The listing builds one solid part. Answer for the finished solid, in the listing's coordinates (mm). Face numbers are marked on the shaded views. A direction names the side the tool comes from. Coordinates: 2 decimals unless noted, no trailing zeros. Write each loop counter-clockwise with the first axis right and the second up, starting at its lowest first coordinate (ties: lowest second). Pieces come first, ordered by that corner, then holes. Notation, with made-up numbers: M 80.25,60 L 124.25,60 A21 ccw 124.25,93 Z; hole C 68,61 d4. An arc over 180 degrees is marked long. Answer as a JSON object with one key per item and string values. Group by question number.
from build123d import *

# Parameters (mm, degrees)
SKETCH_1_W                    = 120
SKETCH_1_H                    = 40
EXTRUDE_1_DEPTH               = 14
SKETCH_2_W                    = 120
SKETCH_2_H                    = 20
CUT_EXTRUDE_1_DEPTH           = 2
HOLE_WIZARD_M12_1_D           = 13.5
HOLE_WIZARD_M12_1_CBORE_D     = 20
HOLE_WIZARD_M12_1_CBORE_DEPTH = 10
FILLET_1_R                    = 20
HOLE_WIZARD_M6_1_D            = 5


with BuildPart() as part:
    # 草图1 → 凸台-拉伸1 (new body)
    with BuildSketch(Plane.XY):
        Rectangle(SKETCH_1_W, SKETCH_1_H)
    extrude(amount=EXTRUDE_1_DEPTH)

    # 草图2 → 切除-拉伸1 (cut)
    with BuildSketch(Plane.XY.offset(14)):
        Rectangle(SKETCH_2_W, SKETCH_2_H)
    extrude(amount=-CUT_EXTRUDE_1_DEPTH, mode=Mode.SUBTRACT)

    # M12 六角头螺栓的柱形沉头孔1 (through all)
    with Locations(Plane.XY.offset(12)):
        with Locations((-35, 0), (35, 0)):
            CounterBoreHole(HOLE_WIZARD_M12_1_D / 2, HOLE_WIZARD_M12_1_CBORE_D / 2, HOLE_WIZARD_M12_1_CBORE_DEPTH)

    # 圆角1
    fillet_1_edges = [part.edges().sort_by_distance(p)[0] for p in [
        (60, 20, 7),
        (60, -20, 7),
        (-60, -20, 7),
        (-60, 20, 7),
    ]]
    fillet(fillet_1_edges, radius=FILLET_1_R - 0.0001)  # a hair under: the kernel refuses the full size

    # M6 螺纹孔1 (through all)
    with Locations(Plane.XY.offset(12)):
        with Locations((0, 0)):
            Hole(HOLE_WIZARD_M6_1_D / 2)


solid = part.part
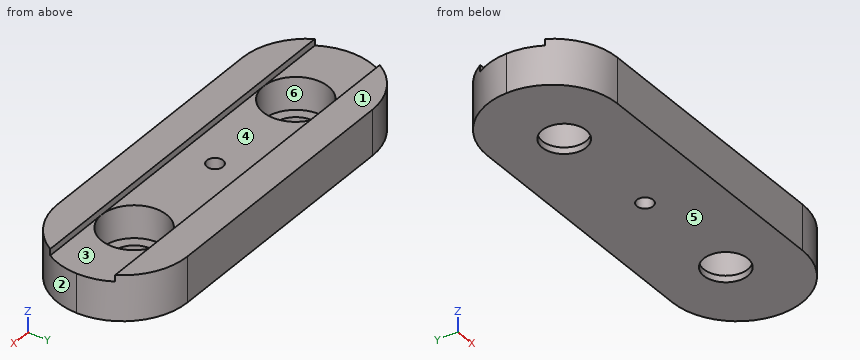
Item 1: Consider L1, parallel to Y at x = 35, z = 1; L2, parallel to X at y = -1, z = 11.25; L3, parallel to Y at x = -35, z = 8.75. Determine where each line is inside the solid, lowest interval first. Write a range as from..to.
Item 2: A cutting plane is placed at C-C, the plane y = 5.5. Write down the section's boundary in (x, z).
Item 3: For a pull along Y with two mould halves and no side action, classify the marked faces 1, 2 and 3 as +Y half, -Y half, draft (parallel to the pull), parting line (faces both ways), or undercut.
Item 4: A cutting plane is placed at B-B, the plane z = 9.5. State how many separate pieces and enclosed holes the cut face has, and give its area (3 significant figures).
Item 5: A tool of negligible diameter and unlimited length cuts with its end or side. For the marked faces 4, 5 and 6, from which of +Z, -Z, +X, -X, +Y, -Y can it reach the whole face along a straight path? Write none if from no direction.
Item 6: A cutting plane is placed at A-A, the plane x = 0. Write down the section's boundary in (y, z), and give its area (3 significant figures).
Item 7: A cutting plane is placed at D-D, the plane x = 18. Write down the section's boundary in (y, z).
Item 8: Flat-ended cylindrical pins translate along their axes: pin 1 Ø4 at (y, z) = (4.5, 7.5) entering from +X; pin 2 Ø16 at (x, y) = (30.5, -2.5) entering from +Z; pin 3 Ø1 at (y, z) = (14, 10) entering from +X; pin 4 Ø17.5 at (x, y) = (-35, 0) entering from +Z. Find the tip coordinate at first contact, or state that the pin passes through.
Answer:
{
 "1": {"L1": "-20..-6.75, 6.75..20", "L2": "-59.97..-44.95, -25.05..-2.29, 2.29..25.05, 44.95..59.97", "L3": "-20..-10, 10..20"},
 "2": {"outline": "M -59.23,0 L -38.91,0 L -38.91,2 L -43.35,2 L -43.35,12 L -59.23,12 Z; M -31.09,0 L 31.09,0 L 31.09,2 L 26.65,2 L 26.65,12 L -26.65,12 L -26.65,2 L -31.09,2 Z; M 38.91,0 L 59.23,0 L 59.23,12 L 43.35,12 L 43.35,2 L 38.91,2 Z"},
 "3": {"face 1": "draft", "face 2": "-Y half", "face 3": "undercut"},
 "4": {"separate pieces": "1", "enclosed holes": "3", "area": "3,810 mm2"},
 "5": {"face 4": "+Z, +X, -X", "face 5": "-Z, +X, -X, +Y, -Y", "face 6": "+Z"},
 "6": {"outline": "M -20,0 L -2.5,0 L -2.5,12 L -10,12 L -10,14 L -20,14 Z; M 2.5,0 L 20,0 L 20,14 L 10,14 L 10,12 L 2.5,12 Z", "area": "460 mm2"},
 "7": {"outline": "M -20,0 L 20,0 L 20,14 L 10,14 L 10,12 L -10,12 L -10,14 L -20,14 Z"},
 "8": {"pin 1": "x = 59.84", "pin 2": "z = 14", "pin 3": "x = 54.76", "pin 4": "z = 2"}
}
